For this review, take the finished solid that the model builds, in its own axes (mm). Face numbers are marked on the shaded views. A direction names the side the tool comes from. Coordinates: 2 decimals unless noted, no trailing zeros. Write each loop counter-clockwise with the first axis right and the second up, starting at its lowest first coordinate (ties: lowest second). Pieces come first, ordered by that corner, then holes.
1) We need section D-D on y = 0.6. Write out the cut boundary in (x, z).
2) Mouldability with a two-part tool opening along Z and no side actions: class the marked faces 1, 2, 3 and 4 as pulls with the +Z half, pulls with the -Z half, needs draft (parallel to the pull), parting line crosses it, or undercut.
3) We need section A-A on y = 3.35. Write out the cut boundary in (x, z), then the cut area to 3 significant figures.
4) We need section C-C on z = 12.5. Write out the cut boundary in (x, y), then the cut area to 3 significant figures.
5) We need section B-B on x = -12.5. Write out the cut boundary in (y, z), then the cut area to 3 significant figures.
6) To check wall thickness, follow line 1 along X through (y, z) = (3.75, -2); line 2 along Z through (x, y) = (-12, 2.9); line 3 along Y through (x, z) = (-14, 5). State the ranges of each line that lie inside material, in increasing order.
7) Insertion check: P1, Ø2.5, axis at x = -12.5, z = 0, coming from the +Y side; P2, Ø4, axis at x = -15.5, z = -1, coming from the -Y side; P3, Ø1, axis at y = 0.5, z = -5, coming from the -X side; P4, Ø2, axis at x = -11.5, y = 1, coming from the +Z side. Each pin has a flat end and moves straight along its axis. Give the tip position at first contact, or say it passes through.
8) For the marked faces 5 and 6, list the 3-axis set-ups (+Z, -Z, +X, -X, +Y, -Y) from which the entire face can be reached by the end or side of a thin tool; tool diameter is ignored.
from build123d import *

# Parameters (mm, degrees)
SKETCH_1_R          = 1.65
EXTRUDE_1_DEPTH     = 4
SKETCH_1_4_R        = 1.65
CUT_EXTRUDE_4_DEPTH = 2
CUT_EXTRUDE_2_DEPTH = 35.597398746
FILLET_1_R          = 0.5


with BuildPart() as part:
    # Sketch 1 → Extrude 1 (new body)
    with BuildSketch(Plane(origin=(0, 0, 0), x_dir=(1, 0, 0), z_dir=(0, 1, 0))):
        with BuildLine():
            ThreePointArc((-10.308655527, 18.24209206), (-13.722071454, 13.722071454), (-18.24209206, 10.308655527))
            ThreePointArc((-18.24209206, 10.308655527), (-24.299735034, 0.079076788), (-18.37973853, -10.230770979))
            ThreePointArc((-18.37973853, -10.230770979), (-13.764731337, -13.764731337), (-10.230770979, -18.37973853))
            ThreePointArc((-10.230770979, -18.37973853), (0, -24.3), (10.230770979, -18.37973853))
            ThreePointArc((10.230770979, -18.37973853), (13.764731337, -13.764731337), (18.37973853, -10.230770979))
            ThreePointArc((18.37973853, -10.230770979), (24.299735034, 0.079076788), (18.24209206, 10.308655527))
            ThreePointArc((18.24209206, 10.308655527), (13.722071454, 13.722071454), (10.308655527, 18.24209206))
            ThreePointArc((10.308655527, 18.24209206), (0, 24.3), (-10.308655527, 18.24209206))
        make_face()
        with Locations(Location((-12.5, 0, 0), (0, 0, 270))):
            Circle(SKETCH_1_R, mode=Mode.SUBTRACT)
        with Locations(Location((0, 12.5, 0), (0, 0, 270))):
            Circle(SKETCH_1_R, mode=Mode.SUBTRACT)
        with Locations(Location((12.5, 0, 0), (0, 0, 270))):
            Circle(SKETCH_1_R, mode=Mode.SUBTRACT)
        with Locations(Location((0, -12.5, 0), (0, 0, 270))):
            Circle(SKETCH_1_R, mode=Mode.SUBTRACT)
    extrude(amount=EXTRUDE_1_DEPTH)

    # Sketch 1_4 → Cut-Extrude 4 (cut)
    with BuildSketch(Plane(origin=(0, 0, 0), x_dir=(1, 0, 0), z_dir=(0, 1, 0))):
        with BuildLine():
            ThreePointArc((15.390040972, -5.02868404), (9.52209065, -9.52209065), (5.02868404, -15.390040972))
            ThreePointArc((5.02868404, -15.390040972), (0, -18.3), (-5.02868404, -15.390040972))
            ThreePointArc((-5.02868404, -15.390040972), (-9.52209065, -9.52209065), (-15.390040972, -5.02868404))
            ThreePointArc((-15.390040972, -5.02868404), (-18.299869762, 0.038868252), (-15.322384233, 5.066966276))
            ThreePointArc((-15.322384233, 5.066966276), (-9.479430767, 9.479430767), (-5.066966276, 15.322384233))
            ThreePointArc((-5.066966276, 15.322384233), (0, 18.3), (5.066966276, 15.322384233))
            ThreePointArc((5.066966276, 15.322384233), (9.479430767, 9.479430767), (15.322384233, 5.066966276))
            ThreePointArc((15.322384233, 5.066966276), (18.299869762, 0.038868252), (15.390040972, -5.02868404))
        make_face()
        with Locations(Location((0, -12.5, 0), (0, 0, 270))):
            Circle(SKETCH_1_4_R, mode=Mode.SUBTRACT)
        with Locations(Location((12.5, 0, 0), (0, 0, 270))):
            Circle(SKETCH_1_4_R, mode=Mode.SUBTRACT)
        with Locations(Location((0, 12.5, 0), (0, 0, 270))):
            Circle(SKETCH_1_4_R, mode=Mode.SUBTRACT)
        with Locations(Location((-12.5, 0, 0), (0, 0, 270))):
            Circle(SKETCH_1_4_R, mode=Mode.SUBTRACT)
    extrude(amount=CUT_EXTRUDE_4_DEPTH, mode=Mode.SUBTRACT)

    # Sketch 3 → Cut-Extrude 2 (cut, through all)
    with BuildSketch(Plane(origin=(0, 4, 0), x_dir=(1, 0, 0), z_dir=(0, 1, 0))):
        with BuildLine():
            Line((6.285747384, 22.486459824), (-0.25936461, 15.94134783))
            Line((-0.25936461, 15.94134783), (3.181980515, 12.499997674))
            Line((3.181980515, 12.499997674), (-3.535538817, 5.782488163))
            Line((-3.535538817, 5.782488163), (1.123471267, 1.123471267))
            Line((1.123471267, 1.123471267), (5.782488163, -3.535538817))
            Line((5.782488163, -3.535538817), (12.499997674, 3.181980515))
            Line((12.499997674, 3.181980515), (15.94134783, -0.25936461))
            Line((15.94134783, -0.25936461), (22.486459824, 6.285747384))
            ThreePointArc((22.486459824, 6.285747384), (20.617437008, 8.564298945), (18.24209206, 10.308655527))
            ThreePointArc((18.24209206, 10.308655527), (13.722071454, 13.722071454), (10.308655527, 18.24209206))
            ThreePointArc((10.308655527, 18.24209206), (8.564298945, 20.617437008), (6.285747384, 22.486459824))
        make_face()
    extrude(amount=-CUT_EXTRUDE_2_DEPTH, mode=Mode.SUBTRACT)

    # Fillet 1
    fillet_1_edges = [part.edges().sort_by_distance(p)[0] for p in [
        (15.94134783, 3, 0.25936461),
        (12.499997674, 3, -3.181980515),
        (5.782488163, 3, 3.535538817),
        (-3.535538817, 3, -5.782488163),
        (3.181980515, 3, -12.499997674),
        (18.010435708, 1, -1.809723268),
        (22.486459824, 2, -6.285747384),
        (1.809723268, 1, -18.010435708),
        (-0.25936461, 3, -15.94134783),
        (6.285747384, 2, -22.486459824),
    ]]
    fillet(fillet_1_edges, radius=FILLET_1_R)


solid = part.part
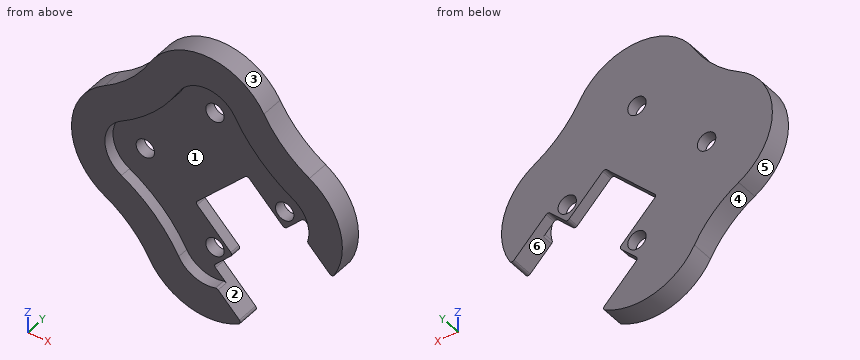
Result:
1. outline: (-18.38, 10.23) arc R11.8 ccw to (-18.24, -10.31) arc R20.5 cw to (-10.31, -18.24) arc R11.8 ccw to (5.72, -22.82) arc R0.5 ccw to (5.83, -22.03) - (2.02, -18.22) arc R0.5 ccw to (1.54, -18.09) arc R5.8 cw to (-5.07, -15.32) arc R26.5 ccw to (-15.32, -5.07) arc R5.8 cw to (-15.39, 5.03) arc R28.1 ccw to (-5.03, 15.39) arc R5.8 cw to (5.03, 15.39) arc R28.1 ccw to (15.39, 5.03) arc R5.8 cw to (18.09, -1.54) arc R0.5 ccw to (18.22, -2.02) - (22.03, -5.83) arc R0.5 ccw to (22.82, -5.72) arc R11.8 ccw to (18.38, 10.23) arc R22.1 cw to (10.23, 18.38) arc R11.8 ccw to (-10.23, 18.38) arc R22.1 cw to start
2. face 1: undercut
2. face 2: undercut
2. face 3: pulls with the +Z half
2. face 4: pulls with the -Z half
3. outline: (-18.38, 10.23) arc R11.8 ccw to (-18.24, -10.31) arc R20.5 cw to (-10.31, -18.24) arc R11.8 ccw to (5.72, -22.82) arc R0.5 ccw to (5.83, -22.03) - (0.09, -16.29) arc R0.5 cw to (0.09, -15.59) - (2.83, -12.85) arc R0.5 ccw to (2.83, -12.15) - (-3.18, -6.14) arc R0.5 cw to (-3.18, -5.43) - (1.12, -1.12) - (5.43, 3.18) arc R0.5 cw to (6.14, 3.18) - (12.15, -2.83) arc R0.5 ccw to (12.85, -2.83) - (15.59, -0.09) arc R0.5 cw to (16.29, -0.09) - (22.03, -5.83) arc R0.5 ccw to (22.82, -5.72) arc R11.8 ccw to (18.38, 10.23) arc R22.1 cw to (10.23, 18.38) arc R11.8 ccw to (-10.23, 18.38) arc R22.1 cw to start; hole circle Ø3.3 at (-12.5, 0); hole circle Ø3.3 at (0, -12.5); hole circle Ø3.3 at (0, 12.5); hole circle Ø3.3 at (12.5, 0)
3. area: 1,170 mm2
4. outline: (-15.14, 0) - (-6.94, 0) - (-6.94, 2) - (-1.65, 2) - (-1.65, 4) - (-15.14, 4) - close; (1.65, 2) - (6.94, 2) - (6.94, 0) - (15.14, 0) - (15.14, 4) - (1.65, 4) - close
4. area: 86.8 mm2
5. outline: (0, -15.06) - (4, -15.06) - (4, -1.65) - (2, -1.65) - (2, -6.88) - (0, -6.88) - close; (0, 6.94) - (2, 6.94) - (2, 1.65) - (4, 1.65) - (4, 15.14) - (0, 15.14) - close
5. area: 86.6 mm2
6. line 1: x = -24.13 to 0.25, 11.32 to 13.68, 18.2 to 24.13
6. line 2: z = -15.68 to -1.57, 1.57 to 15.76
6. line 3: y = 2 to 4
7. P1: passes through
7. P2: stops at y = 2
7. P3: stops at x = -23.41
7. P4: stops at z = 17.92
8. face 5: -X, +Y, -Y
8. face 6: -Z, +Y, -Y
